Geometry: final body of the model. Coordinates: model frame, mm. Face numbers are marked on the shaded views. A direction names the side the tool comes from. Give positions to 0.01 mm unless a question says otherwise; leave off trailing zeros. Order: outer loops, then holes, each group sorted by start corner. A loop starts at its lowest first (then second) coordinate and runs counter-clockwise, first axis right, second up. Notation, with made-up numbers: M -18.5,72 L 36.5,72 A24 ccw 36.5,103 Z; hole C -16,38.25 d9. An arc over 180 degrees is marked long. Write item = value, one per line. Start each with the question number.
from build123d import *

# Parameters (mm, degrees)
SKETCH1_W               = 33
SKETCH1_H               = 17.983376384
BOSS_EXTRUDE1_DEPTH     = 9
SKETCH4_W               = 5
SKETCH4_H               = 12.3
BOSS_EXTRUDE2_DEPTH     = 5
CHAMFER1_SIZE           = 13
CHAMFER1_SIZE_2         = 12.3
SKETCH2_R               = 1.575
CUT_EXTRUDE1_DEPTH      = 29.404057044
CUT_EXTRUDE2_DEPTH      = 23.458638795
CUT_EXTRUDE2_DEPTH_BACK = 3.2
SKETCH3_R               = 3.05
CUT_EXTRUDE3_REACH      = 34.394
SKETCH5_R               = 0.975
SKETCH6_W               = 33
SKETCH6_H               = 9
BOSS_EXTRUDE3_DEPTH     = 9.9
CUT_EXTRUDE4_START      = 2
CUT_EXTRUDE4_DEPTH      = 8
SKETCH8_R               = 1.45
CUT_EXTRUDE5_DEPTH      = 10
SKETCH9_R               = 1.45
BOSS_EXTRUDE4_DEPTH     = 5
SKETCH10_W              = 1.52
SKETCH10_H              = 9.9
CUT_EXTRUDE6_DEPTH      = 9
FILLET1_R               = 1.3


with BuildPart() as part:
    # Sketch1 → Boss-Extrude1 (new body)
    with BuildSketch(Plane.XY):
        Rectangle(SKETCH1_W, SKETCH1_H)
    extrude(amount=BOSS_EXTRUDE1_DEPTH)

    # Sketch4 → Boss-Extrude2 (add)
    with BuildSketch(Plane(origin=(0, 8.991688192, 0), x_dir=(1, 0, 0), z_dir=(0, 1, 0))):
        with Locations((-14, -15.15)):
            Rectangle(SKETCH4_W, SKETCH4_H)
        with Locations((14, -15.15)):
            Rectangle(SKETCH4_W, SKETCH4_H)
    extrude(amount=-BOSS_EXTRUDE2_DEPTH)

    # Chamfer1
    # the kernel refuses this chamfer: 13, 12.3 mm, written as the material it adds along each edge
    with BuildSketch(Plane(origin=(-16.5, 3.991688192, 9), x_dir=(0, -0.9996433463604261, -0.02670543160724426), z_dir=(1, 0, 0))) as chamfer1_piece_1_section:
        Polygon((CHAMFER1_SIZE * 0.99964334636, -CHAMFER1_SIZE * 0.0267054316072), (-CHAMFER1_SIZE_2 * 0.0267054316072, -CHAMFER1_SIZE_2 * 0.99964334636), (0, 0), align=None)
    chamfer1_piece_1 = extrude(amount=5, mode=Mode.PRIVATE)
    chamfer1_piece_1 = split(chamfer1_piece_1, bisect_by=Plane(origin=(-14, -8.991688192, 13.04185716), z_dir=(0, 1, 0)), keep=Keep.TOP, mode=Mode.PRIVATE)
    chamfer1_piece_1 = split(chamfer1_piece_1, bisect_by=Plane(origin=(-14, -0.292838715, 21.3), z_dir=(0, 0, -1)), keep=Keep.TOP, mode=Mode.PRIVATE)
    add(chamfer1_piece_1)
    with BuildSketch(Plane(origin=(-16.5, 3.991688192, 9), x_dir=(0, -0.9996433463604261, -0.02670543160724426), z_dir=(1, 0, 0))) as chamfer1_piece_2_section:
        Polygon((CHAMFER1_SIZE * 0.99964334636, -CHAMFER1_SIZE * 0.0267054316072), (-CHAMFER1_SIZE_2 * 0.0267054316072, -CHAMFER1_SIZE_2 * 0.99964334636), (0, 0), align=None)
    chamfer1_piece_2 = extrude(amount=38.456243217, mode=Mode.PRIVATE)
    chamfer1_piece_2 = split(chamfer1_piece_2, bisect_by=Plane(origin=(14, -8.991688192, 13.04185716), z_dir=(0, 1, 0)), keep=Keep.TOP, mode=Mode.PRIVATE)
    chamfer1_piece_2 = split(chamfer1_piece_2, bisect_by=Plane(origin=(16.5, -0.292838715, 13.04185716), z_dir=(-1, 0, 0)), keep=Keep.TOP, mode=Mode.PRIVATE)
    chamfer1_piece_2 = split(chamfer1_piece_2, bisect_by=Plane(origin=(11.5, -0.292838715, 13.04185716), z_dir=(1, 0, 0)), keep=Keep.TOP, mode=Mode.PRIVATE)
    chamfer1_piece_2 = split(chamfer1_piece_2, bisect_by=Plane(origin=(14, -0.292838715, 21.3), z_dir=(0, 0, -1)), keep=Keep.TOP, mode=Mode.PRIVATE)
    add(chamfer1_piece_2)
    with BuildSketch(Plane(origin=(16.5, 3.991688192, 9), x_dir=(0, -0.9996433463604261, -0.02670543160724426), z_dir=(-1, 0, 0))) as chamfer1_piece_3_section:
        Polygon((CHAMFER1_SIZE * 0.99964334636, CHAMFER1_SIZE * 0.0267054316072), (-CHAMFER1_SIZE_2 * 0.0267054316072, CHAMFER1_SIZE_2 * 0.99964334636), (0, 0), align=None)
    chamfer1_piece_3 = extrude(amount=5, mode=Mode.PRIVATE)
    chamfer1_piece_3 = split(chamfer1_piece_3, bisect_by=Plane(origin=(14, -8.991688192, 13.04185716), z_dir=(0, 1, 0)), keep=Keep.TOP, mode=Mode.PRIVATE)
    chamfer1_piece_3 = split(chamfer1_piece_3, bisect_by=Plane(origin=(14, -0.292838715, 21.3), z_dir=(0, 0, -1)), keep=Keep.TOP, mode=Mode.PRIVATE)
    add(chamfer1_piece_3)
    with BuildSketch(Plane(origin=(16.5, 3.991688192, 9), x_dir=(0, -0.9996433463604261, -0.02670543160724426), z_dir=(-1, 0, 0))) as chamfer1_piece_4_section:
        Polygon((CHAMFER1_SIZE * 0.99964334636, CHAMFER1_SIZE * 0.0267054316072), (-CHAMFER1_SIZE_2 * 0.0267054316072, CHAMFER1_SIZE_2 * 0.99964334636), (0, 0), align=None)
    chamfer1_piece_4 = extrude(amount=38.456243217, mode=Mode.PRIVATE)
    chamfer1_piece_4 = split(chamfer1_piece_4, bisect_by=Plane(origin=(-14, -8.991688192, 13.04185716), z_dir=(0, 1, 0)), keep=Keep.TOP, mode=Mode.PRIVATE)
    chamfer1_piece_4 = split(chamfer1_piece_4, bisect_by=Plane(origin=(-16.5, -0.292838715, 13.04185716), z_dir=(1, 0, 0)), keep=Keep.TOP, mode=Mode.PRIVATE)
    chamfer1_piece_4 = split(chamfer1_piece_4, bisect_by=Plane(origin=(-14, -0.292838715, 21.3), z_dir=(0, 0, -1)), keep=Keep.TOP, mode=Mode.PRIVATE)
    chamfer1_piece_4 = split(chamfer1_piece_4, bisect_by=Plane(origin=(-11.5, -0.292838715, 13.04185716), z_dir=(-1, 0, 0)), keep=Keep.TOP, mode=Mode.PRIVATE)
    add(chamfer1_piece_4)

    # Sketch2 → Cut-Extrude1 (cut, through all)
    with BuildSketch(Plane(origin=(0, 0, 0), x_dir=(-1, 0, 0), z_dir=(0, 0, -1))):
        with Locations((-2, 0)):
            Circle(SKETCH2_R)
        with Locations((-10, 0)):
            Circle(SKETCH2_R)
    extrude(amount=-CUT_EXTRUDE1_DEPTH, mode=Mode.SUBTRACT)

    # Sketch3 → Cut-Extrude2 (cut, two sides: drawn at the far end of the back side and taken through both)
    with BuildSketch(Plane.XY.offset(9).offset(-CUT_EXTRUDE2_DEPTH_BACK)):
        with Locations((2, 0)):
            Circle(SKETCH3_R)
        with Locations(Location((10, 0, 0), (0, 0, 60.540825088))):
            Circle(SKETCH3_R)
    extrude(amount=CUT_EXTRUDE2_DEPTH + CUT_EXTRUDE2_DEPTH_BACK, mode=Mode.SUBTRACT)

    # Cut-Extrude3: up to this plane
    cut_extrude3_end = Plane(origin=(0, -9.008311808, 9), z_dir=(0, 0.6872795500600087, -0.726393020388627))
    # Sketch5 → Cut-Extrude3 (cut, up to the surface)
    with BuildSketch(Plane(origin=(0, 8.991688192, 0), x_dir=(1, 0, 0), z_dir=(0, 1, 0)), mode=Mode.PRIVATE) as cut_extrude3_sk1:
        with Locations(Location((-14, -15.15, 0), (0, 0, 180))):
            Circle(SKETCH5_R)
    cut_extrude3_tool1 = split(extrude(cut_extrude3_sk1.sketch, amount=-CUT_EXTRUDE3_REACH, mode=Mode.PRIVATE), bisect_by=cut_extrude3_end, keep=Keep.BOTH, mode=Mode.PRIVATE)
    add(cut_extrude3_tool1.solids().sort_by_distance((-14, 8.991688, 15.15))[0], mode=Mode.SUBTRACT)
    # Sketch5 → Cut-Extrude3 (cut, up to the surface)
    with BuildSketch(Plane(origin=(0, 8.991688192, 0), x_dir=(1, 0, 0), z_dir=(0, 1, 0)), mode=Mode.PRIVATE) as cut_extrude3_sk2:
        with Locations(Location((14, -15.15, 0), (0, 0, 270))):
            Circle(SKETCH5_R)
    cut_extrude3_tool2 = split(extrude(cut_extrude3_sk2.sketch, amount=-CUT_EXTRUDE3_REACH, mode=Mode.PRIVATE), bisect_by=cut_extrude3_end, keep=Keep.BOTH, mode=Mode.PRIVATE)
    add(cut_extrude3_tool2.solids().sort_by_distance((14, 8.991688, 15.15))[0], mode=Mode.SUBTRACT)

    # Sketch6 → Boss-Extrude3 (add)
    with BuildSketch(Plane(origin=(0, 8.991688192, 0), x_dir=(1, 0, 0), z_dir=(0, 1, 0))):
        with Locations((0, -4.5)):
            Rectangle(SKETCH6_W, SKETCH6_H)
    extrude(amount=BOSS_EXTRUDE3_DEPTH)

    # Sketch7 → Cut-Extrude4 (cut)
    with BuildSketch(Plane.XY.offset(9).offset(CUT_EXTRUDE4_START)):
        Polygon((11.5, -2.655654345), (11.5, -5.508311808), (16.5, -5.508311808), (16.5, -0.508311808), (11.5, -0.508311808), align=None)
        Polygon((16.5, -5.508311808), (11.5, -5.508311808), (11.5, -8.991688192), (11.5, -10.104288395), (16.5, -10.104288395), align=None)
    extrude(amount=CUT_EXTRUDE4_DEPTH, mode=Mode.SUBTRACT)

    # Sketch8 → Cut-Extrude5 (cut)
    with BuildSketch(Plane(origin=(0, 18.891688192, 0), x_dir=(1, 0, 0), z_dir=(0, 1, 0))):
        with Locations(Location((-11.53, -4.9, 0), (0, 0, 180))):
            Circle(SKETCH8_R)
    cut_extrude5 = extrude(amount=-CUT_EXTRUDE5_DEPTH, mode=Mode.SUBTRACT)

    # Sketch9 → Boss-Extrude4 (add)
    with BuildSketch(Plane(origin=(0, 18.891688192, 0), x_dir=(1, 0, 0), z_dir=(0, 1, 0))):
        with BuildLine():
            Line((-11.53, 0), (-1.44116457, 0))
            ThreePointArc((-1.44116457, 0), (3.05883543, -4.5), (-1.44116457, -9))
            Line((-1.44116457, -9), (-11.53, -9))
            ThreePointArc((-11.53, -9), (-16.03, -4.5), (-11.53, 0))
        make_face()
        with Locations(Location((-11.53, -4.9, 0), (0, 0, 180))):
            Circle(SKETCH9_R, mode=Mode.SUBTRACT)
    boss_extrude4 = extrude(amount=-BOSS_EXTRUDE4_DEPTH)

    # Mirror1: Cut-Extrude5, Boss-Extrude4 across plane
    add(cut_extrude5.mirror(Plane(origin=(6, 0, 0), x_dir=(0, 0, 1), z_dir=(1, 0, 0))), mode=Mode.SUBTRACT)
    add(boss_extrude4.mirror(Plane(origin=(6, 0, 0), x_dir=(0, 0, 1), z_dir=(1, 0, 0))))

    # Sketch10 → Cut-Extrude6 (cut)
    with BuildSketch(Plane(origin=(0, 0, 0), x_dir=(-1, 0, 0), z_dir=(0, 0, -1))):
        with Locations((15.74, 13.941688192)):
            Rectangle(SKETCH10_W, SKETCH10_H)
    extrude(amount=-CUT_EXTRUDE6_DEPTH, mode=Mode.SUBTRACT)

    # Fillet1
    fillet1_edges = [part.edges().sort_by_distance(p)[0] for p in [
        (-14.98, 8.991688192, 4.5),
    ]]
    fillet(fillet1_edges, radius=FILLET1_R)


solid = part.part
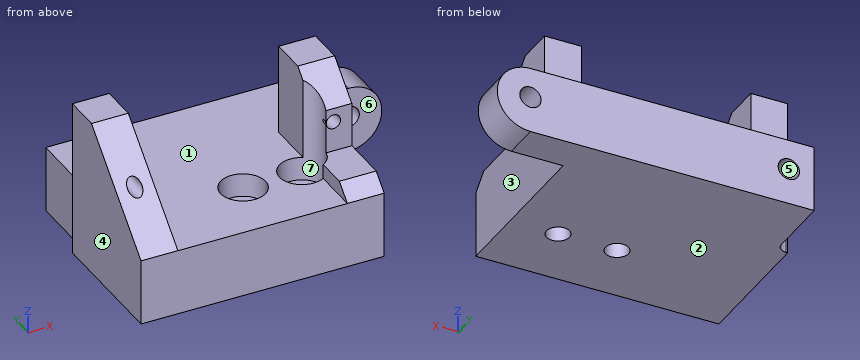
1) Cut plane A-A (y = 0). Return loops of the section in (x, z) (3 decimals), plus the area to 3 significant figures.
2) Cut plane D-D (y = 5.75). Return loops of the section in (x, z) (3 decimals), plus the area to 3 significant figures.
3) Access query for the marked faces 5, 6 and 7. Directions: +Z, -Z, +X, -X, +Y, -Y. A direction counts if a zero-diameter tool reaches every point of the face in a straight line with its end or side. Return the directions, or none.
4) Ray query, L1, parallel to Z at x = 23.53, y = 15.3; L2, parallel to X at y = 2.5, z = 15.15 (3 decimals); L3, parallel to X at y = 4.5, z = 10. Return the intervals inside material, ascending.
5) Pin query (flat end, axial travel): pin 1 Ø2 at (x, z) = (15.5, 9.5) entering from -Y; pin 2 Ø12 at (x, z) = (22, 18) entering from +Y; pin 3 Ø6.5 at (x, y) = (3, 0.5) entering from +Z; pin 4 Ø12 at (x, z) = (11, 15.5) entering from -Y. Return the tip coordinate at first contact, or that it passes through.
6) Cut plane C-C (z = 19.5). Return loops of the section in (x, y).
7) Draft query along X for the marked faces 1, 2, 3 and 4. Return one class per face: pulls with the +X half, pulls with the -X half, needs draft (parallel to the pull), parting line crosses it, or undercut.
8) Cut plane B-B (x = 10). Return loops of the section in (y, z) (3 decimals), plus the area to 3 significant figures.
Reply:
q1.outline = M -16.5,0 L 0.425,0 L 0.425,5.8 L -1.05,5.8 L -1.05,9 L -11.5,9 L -11.5,17.523 L -16.5,17.523 Z; M 3.575,0 L 8.425,0 L 8.425,5.8 L 6.95,5.8 L 6.95,9 L 5.05,9 L 5.05,5.8 L 3.575,5.8 Z; M 11.575,0 L 16.5,0 L 16.5,17.523 L 13.05,17.523 L 13.05,15.369 A0.975 cw long 13.05,14.931 L 13.05,5.8 L 11.575,5.8 Z; hole C -14,15.15 d1.95
q1.area = 287 mm²
q2.outline = M -16.5,0 L 16.5,0 L 16.5,21.3 L 11.5,21.3 L 11.5,9 L -11.5,9 L -11.5,21.3 L -16.5,21.3 Z; hole C -14,15.15 d1.95; hole C 14,15.15 d1.95
q2.area = 414 mm²
q3.face_5 = +Y
q3.face_6 = +Z, -Z, +X, -Y
q3.face_7 = +Z
q4.L1 = 0 to 3.45, 6.35 to 9
q4.L2 = -16.5 to -14.975, -13.025 to -11.5, 11.747 to 13.025, 14.975 to 16.5
q4.L3 = -16.5 to -11.5, 11.5 to 16.5
q5.pin_1 = -8.99
q5.pin_2 = 8.99
q5.pin_3 = 9
q5.pin_4 = -8.46
q6.outline = M -16.5,2.09 L -11.5,2.09 L -11.5,8.99 L -16.5,8.99 Z; M 11.5,2.66 A3.05 cw 12.22,2.09 L 16.5,2.09 L 16.5,8.99 L 11.5,8.99 Z
q7.face_1 = undercut
q7.face_2 = needs draft
q7.face_3 = pulls with the +X half
q7.face_4 = pulls with the -X half
q8.outline = M -8.992,0 L -1.575,0 L -1.575,5.8 L -3.05,5.8 L -3.05,9 L -8.992,9 Z; M 1.575,0 L 18.892,0 L 18.892,9 L 3.05,9 L 3.05,5.8 L 1.575,5.8 Z
q8.area = 213 mm²
